Here's how the part is built. I have some questions about the finished solid (model axes, mm). Face numbers are marked on the shaded views. A direction names the side the tool comes from. Round coordinates to 2 decimals unless told otherwise and drop trailing zeros. Write each loop counter-clockwise with the first axis right and the second up, starting at its lowest first coordinate (ties: lowest second). Pieces come first, ordered by that corner, then holes. Notation, with made-up numbers: (14, 66.25) - (46, 66.25) arc R30 cw to (46, 91.25) - close; hole circle Ø7 at (20, 66). An arc over 180 degrees is marked (long way). One line per item, written item: value. Start each with the question number.
Item 1: Imagine slicing it at A-A, the plane x = -59.5. Please give me the cut outline in (y, z), then the cut area to 3 significant figures.
Item 2: For the marked faces 1, 2 and 3, which set-ups out of +Z, -Z, +X, -X, +Y, -Y let a thin tool reach every point of the face, with its end or its side?
Item 3: Imagine slicing it at C-C, the plane z = 17. Please give me the cut outline in (x, y) (3 decimals).
Item 4: Imagine slicing it at D-D, the plane y = -4.5. Please give me the cut outline in (x, z).
Item 5: If I drill on line 1 (Y direction, x = -64, z = 19); line 2 (Z direction, x = -30, y = -4); line 3 (Y direction, x = -56.5, z = 30), over which ranges is the centre line in solid material (lowest first)?
Item 6: For P1, Ø8, axis at x = -45, y = -31.5, coming from the +Z side; P2, Ø6, axis at x = -62.5, z = 20, coming from the +Y side; P3, Ø1.5, axis at x = -57.5, z = 34.5, coming from the -Y side; P4, Ø1.5, axis at x = -40.5, y = -8, coming from the +Z side, each with a flat end and sliding along its axis, tell me the tip position at first contact or that it passes through.
Item 7: Thinking about a two-plate mould opening in X: for the marked faces 4, 5 and 6, which applies, released by +X, released by -X, zero draft, split by the parting line, or undercut?
Item 8: Imagine slicing it at B-B, the plane y = -26.5. Please give me the cut outline in (x, z).
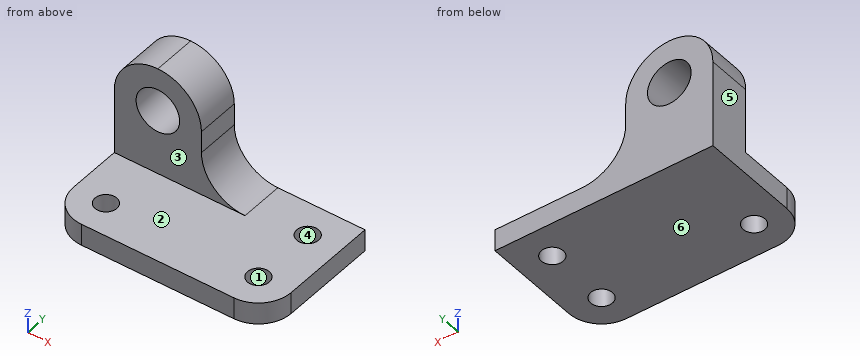
```python
from build123d import *

# Parameters (mm, degrees)
F1_DEPTH  = 38.1
F2_W      = 38.1
F2_H      = 31.75
F3_DEPTH  = 25.4
F4_R      = 3.175
F5_DEPTH  = 25.4
F6_R      = 3.175
F7_DEPTH  = 25.4
F8_R      = 6.35
F9_DEPTH  = 25.4
F11_DEPTH = 25.4


with BuildPart() as f1:
    # F0 (on Front) → F1 (new body)
    with BuildSketch(Plane.XZ):
        Polygon((-35.522558, 52.933332), (-73.622558, 52.933332), (-73.622558, 14.833332), (-10.122558, 14.833332), (-10.122558, 21.183332), (-35.522558, 21.183332), align=None)
    extrude(amount=F1_DEPTH)

    # F2 (on face) → F3 (cut)
    with BuildSketch(Plane.XZ.offset(38.1)):
        with Locations((-54.572558, 37.058332)):
            Rectangle(F2_W, F2_H)
    extrude(amount=-F3_DEPTH, mode=Mode.SUBTRACT)

    # F4 (on face) → F5 (cut)
    with BuildSketch(Plane.XY.offset(21.183332)):
        with Locations((-19.647558, -28.575)):
            Circle(F4_R)
        with Locations((-64.097558, -28.575)):
            Circle(F4_R)
        with BuildLine():
            Line((-73.622558, -38.1), (-64.097558, -38.1))
            ThreePointArc((-64.097558, -38.1), (-70.83275, -35.310192), (-73.622558, -28.575))
            Line((-73.622558, -28.575), (-73.622558, -38.1))
        make_face()
        with BuildLine():
            ThreePointArc((-10.122558, -28.575), (-12.912366, -35.310192), (-19.647558, -38.1))
            Line((-19.647558, -38.1), (-10.122558, -38.1))
            Line((-10.122558, -38.1), (-10.122558, -28.575))
        make_face()
    extrude(amount=-F5_DEPTH, mode=Mode.SUBTRACT)

    # F6 (on face) → F7 (cut)
    with BuildSketch(Plane.XY.offset(21.183332)):
        with Locations((-19.647558, -9.525)):
            Circle(F6_R)
    extrude(amount=-F7_DEPTH, mode=Mode.SUBTRACT)

    # F8 (on face) → F9 (cut)
    with BuildSketch(Plane.XZ.offset(12.7)):
        with Locations((-60.922558, 40.233332)):
            Circle(F8_R)
    extrude(amount=-F9_DEPTH, mode=Mode.SUBTRACT)

    # F10 (on face) → F11 (cut)
    with BuildSketch(Plane.XZ.offset(12.7)):
        with BuildLine():
            ThreePointArc((-60.922558, 52.933332), (-51.942302, 49.213588), (-48.222558, 40.233332))
            Line((-48.222558, 40.233332), (-48.222558, 33.883332))
            ThreePointArc((-48.222558, 33.883332), (-44.502814, 24.903076), (-35.522558, 21.183332))
            Line((-35.522558, 21.183332), (-35.522558, 52.933332))
            Line((-35.522558, 52.933332), (-60.922558, 52.933332))
        make_face()
        with BuildLine():
            ThreePointArc((-73.622558, 40.233332), (-69.902814, 49.213588), (-60.922558, 52.933332))
            Line((-60.922558, 52.933332), (-73.622558, 52.933332))
            Line((-73.622558, 52.933332), (-73.622558, 40.233332))
        make_face()
    extrude(amount=-F11_DEPTH, mode=Mode.SUBTRACT)


solid = f1.part
```
Values follow:
1. outline: (-38.1, 14.83) - (0, 14.83) - (0, 34.04) - (-12.7, 34.04) - (-12.7, 21.18) - (-38.1, 21.18) - close; (-12.7, 46.42) - (0, 46.42) - (0, 52.85) - (-12.7, 52.85) - close
1. area: 487 mm^2
2. face 1: +Z, -Z
2. face 2: +Z, +X, -Y
2. face 3: +Z, +X, -X, -Y
3. outline: (-73.623, -28.575) arc R9.525 ccw to (-64.098, -38.1) - (-19.648, -38.1) arc R9.525 ccw to (-10.123, -28.575) - (-10.123, 0) - (-73.623, 0) - close; hole circle Ø6.35 at (-64.098, -28.575); hole circle Ø6.35 at (-19.648, -28.575); hole circle Ø6.35 at (-19.648, -9.525)
4. outline: (-73.62, 14.83) - (-10.12, 14.83) - (-10.12, 21.18) - (-35.52, 21.18) arc R12.7 cw to (-48.22, 33.88) - (-48.22, 40.23) arc R12.7 ccw to (-73.62, 40.23) - close; hole circle Ø12.7 at (-60.92, 40.23)
5. line 1: y = -38.1 to -31.75, -25.4 to 0
5. line 2: z = 14.83 to 21.18
5. line 3: y = -12.7 to 0
6. P1: stops at z = 21.18
6. P2: stops at y = 0
6. P3: stops at y = -12.7
6. P4: stops at z = 22.55
7. face 4: undercut
7. face 5: released by -X
7. face 6: zero draft
8. outline: (-73.62, 14.83) - (-66.5, 14.83) - (-66.5, 21.18) - (-73.62, 21.18) - close; (-61.69, 14.83) - (-22.05, 14.83) - (-22.05, 21.18) - (-61.69, 21.18) - close; (-17.24, 14.83) - (-10.12, 14.83) - (-10.12, 21.18) - (-17.24, 21.18) - close
